Autodesk Inventor part; units mm, degrees
ref_plane "Work Plane1" through (0, 16, 0) normal (0, 1, 0) x (1, 0, 0)
ref_plane "YZ Plane" through (0, 0, 0) normal (1, 0, 0) x (0, 1, 0)
ref_plane "XZ Plane" through (0, 0, 0) normal (0, 1, 0) x (-1, 0, 0)
sketch "Sketch1" plane through (0, 0, 0) normal (0, 1, 0) x (-1, 0, 0)
  line L0 (-35, 10) -> (35, 10)
  line L1 (35, 10) -> (35, -10)
  line L2 (35, -10) -> (-35, -10)
  line L3 (-35, -10) -> (-35, 10)
  line L4 (-35, 10) -> (35, -10) construction
  line L5 (35, 10) -> (-35, -10) construction
  line L6 (0, 0) -> (25, 0)
  line L7 (0, 0) -> (-25, 0)
  circle A0 centre (25, 0) radius 1.5
  circle A1 centre (-25, 0) radius 1.5
  circle A2 centre (0, 0) radius 1.5
  dimension "d0" = 70
  dimension "d1" = 20
  dimension "d2" = 25
  dimension "d3" = 25
  dimension "d4" = 3
  dimension "d5" = 3
  dimension "d8" = 3
extrude "Extrusion1" add sketch "Sketch1" along normal blind 20
sketch "Sketch2" plane through (0, 20, 0) normal (0, 1, 0) x (1, 0, 0)
  circle A0 centre (0, 0) radius 1.5
  circle A1 centre (25, 0) radius 1.5
  circle A2 centre (-25, 0) radius 1.5
  line L0 (-35, -10) -> (35, -10)
  line L1 (35, -10) -> (35, 10)
  line L2 (35, 10) -> (-35, 10)
  line L3 (-35, 10) -> (-35, -10)
  line L4 (-35, 10) -> (-35, -10)
  line L5 (-35, -10) -> (-55, -10)
  line L6 (-55, -10) -> (-55, -2)
  line L7 (-55, -2) -> (-35, -2)
  line L8 (-35, -2) -> (-35, -10)
  line L9 (35, -10) -> (55, -10)
  line L10 (55, -10) -> (55, -2)
  line L11 (55, -2) -> (35, -2)
  line L12 (35, -2) -> (35, -10)
  dimension "d9" = 20
  dimension "d10" = 8
  dimension "d11" = 20
  dimension "d12" = 8
extrude "Extrusion2" add sketch "Sketch2" against normal up to surface (20 mm away) contours L5 L6 L7 L3 | L1 L11 L10 L9
ref_plane "Work Plane1" through (0, 16, 0) normal (0, 1, 0) x (1, 0, 0)
sketch "Sketch3" plane through (0, 16, 0) normal (0, 1, 0) x (1, 0, 0)
  circle A0 centre (0, 0) radius 1.5 construction
  circle A1 centre (25, 0) radius 1.5 construction
  circle A2 centre (-25, 0) radius 1.5 construction
  line L0 (-55, -10) -> (55, -10) construction
  line L1 (55, -10) -> (55, -2) construction
  line L2 (55, -2) -> (35, -2) construction
  line L3 (35, -2) -> (35, 10) construction
  line L4 (35, 10) -> (-35, 10) construction
  line L5 (-35, 10) -> (-35, -2) construction
  line L6 (-35, -2) -> (-55, -2) construction
  line L7 (-55, -2) -> (-55, -10) construction
  circle A3 centre (-25, 0) radius 1.5 construction
  line L8 (-25, 0) -> (-27.6, 0) construction
  line L9 (-27.6, 1.5011) -> (-25, 3.0022)
  line L10 (-25, 3.0022) -> (-22.4, 1.5011)
  line L11 (-22.4, 1.5011) -> (-22.4, -1.5011)
  line L12 (-22.4, -1.5011) -> (-25, -3.0022)
  line L13 (-25, -3.0022) -> (-27.6, -1.5011)
  line L14 (-27.6, -1.5011) -> (-27.6, 1.5011)
  line L15 (-35, 10) -> (35, 10)
  line L16 (-27.6, 1.5011) -> (-22.4, 1.5011)
  line L17 (-22.4, 1.5011) -> (-22.4, 10)
  line L18 (-22.4, 10) -> (-27.6, 10)
  line L19 (-27.6, 10) -> (-27.6, 1.5011)
  dimension "d17" = 2.6
extrude "Extrusion3" cut sketch "Sketch3" against normal blind 3
pattern_linear "Rectangular Pattern1" count 3 spacing 25 along (1, 0, 0) of "Extrusion3"
fillet "Fillet1" radius 2 8 edges at (0, 0, 10) (0, 0, -10) (-35, 0, -4) (-45, 0, 2) (-55, 0, 6) (35, 0, -4) (45, 0, 2) (55, 0, 6)
fillet "Fillet1" radius 4 2 edges at (55, 10, 10) (-55, 10, 10)
properties part number "foot_front"
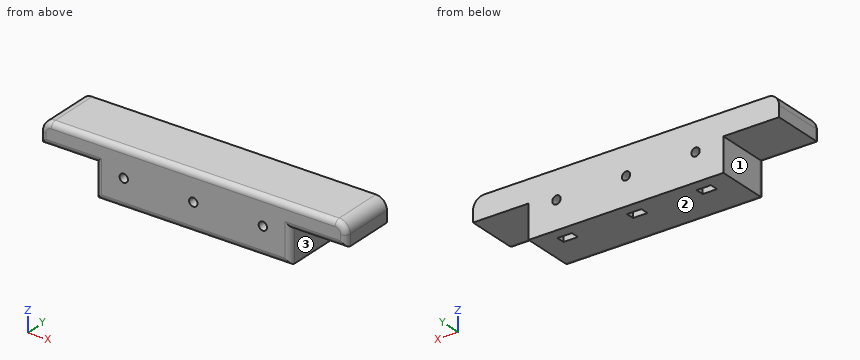
The listing builds one solid part. Answer for the finished solid, in the listing's coordinates (mm). Face numbers are marked on the shaded views. A direction names the side the tool comes from. Round coordinates to 2 decimals unless told otherwise and drop trailing zeros. Write each loop counter-clockwise with the first axis right and the second up, starting at its lowest first coordinate (ties: lowest second). Pieces come first, ordered by that corner, then holes. Notation, with made-up numbers: (14.5, -10) - (32.5, -10) arc R26 cw to (32.5, 4) - close; hole circle Ø4 at (-8.5, 16). An arc over 180 degrees is marked (long way). Use one line per item in the form item = value. Start each with the question number.
Item 1: Find the intervals of material crossed by line 1 (X direction, y = 18.3, z = 0); line 2 (X direction, y = 14.25, z = -3); line 3 (Y direction, x = 22.5, z = -1.5), in increasing order. Write a range as [from, to].
Item 2: A tool of negligible diameter and unlimited length cuts with its end or side. For the marked faces 1, 2 and 3, from which of +Z, -Z, +X, -X, +Y, -Y can it reach the whole face along a straight path? Write none if from no direction.
Item 3: A cutting plane is placed at A-A (z = -3.5). Write down the section's boundary in (x, y).
Item 4: Flat-ended cylindrical pins translate along their axes: pin 1 Ø0.9 at (y, z) = (14, -2.5) entering from +X; pin 2 Ø1.8 at (x, z) = (0, 0) entering from +Y; pin 3 Ø2 at (y, z) = (12.5, -8) entering from -X. Find the tip coordinate at first contact, or state that the pin passes through.
Item 5: A cutting plane is placed at C-C (x = 47). Write down the section's boundary in (y, z), plus the area to 3 significant figures.
Item 6: A cutting plane is placed at B-B (y = 17). Write down the section's boundary in (x, z).
The answers:
q1.line_1 = [-35, -26.5], [-23.5, -1.5], [1.5, 23.5], [26.5, 35]
q1.line_2 = [-35, -27.6], [-22.4, -2.6], [2.6, 22.4], [27.6, 35]
q1.line_3 = [0, 13], [16, 20]
q2.face_1 = -Z, -X, +Y, -Y
q2.face_2 = -Z, +X, -X, +Y, -Y
q2.face_3 = -Z, +X, +Y, -Y
q3.outline = (-35, 2) arc R2 ccw to (-33, 0) - (33, 0) arc R2 ccw to (35, 2) - (35, 20) - (-35, 20) - close; hole (-27.6, 13) - (-22.4, 13) - (-22.4, 16) - (-27.6, 16) - close; hole (-2.6, 13) - (2.6, 13) - (2.6, 16) - (-2.6, 16) - close; hole (22.4, 13) - (27.6, 13) - (27.6, 16) - (22.4, 16) - close
q4.pin_1 = 35
q4.pin_2 = through
q4.pin_3 = -35
q5.outline = (0, 4) arc R2 ccw to (2, 2) - (20, 2) - (20, 10) - (2, 10) arc R2 ccw to (0, 8) - close
q5.area = 158 mm^2
q6.outline = (-55, 2) - (-35, 2) - (-35, -10) - (35, -10) - (35, 2) - (55, 2) - (55, 6) arc R4 ccw to (51, 10) - (-51, 10) arc R4 ccw to (-55, 6) - close; hole circle Ø3 at (-25, 0); hole circle Ø3 at (0, 0); hole circle Ø3 at (25, 0)
